Could you check a few things on this drawing? It's one solid part, dimensions in mm from its lowest x, y, z. Give positions to 0.01 mm unless a question says otherwise; leave off trailing zeros. Order: outer loops, then holes, each group sorted by start corner. A loop starts at its lowest first (then second) coordinate and runs counter-clockwise, first axis right, second up. Notation, with made-up numbers: (83.25, -6.75) - (100.25, -6.75) arc R30 ccw to (100.25, 28.25) - close; hole circle Ø9 at (60.5, 65). An arc over 180 degrees is marked (long way). Answer as CSV lines item,"result".
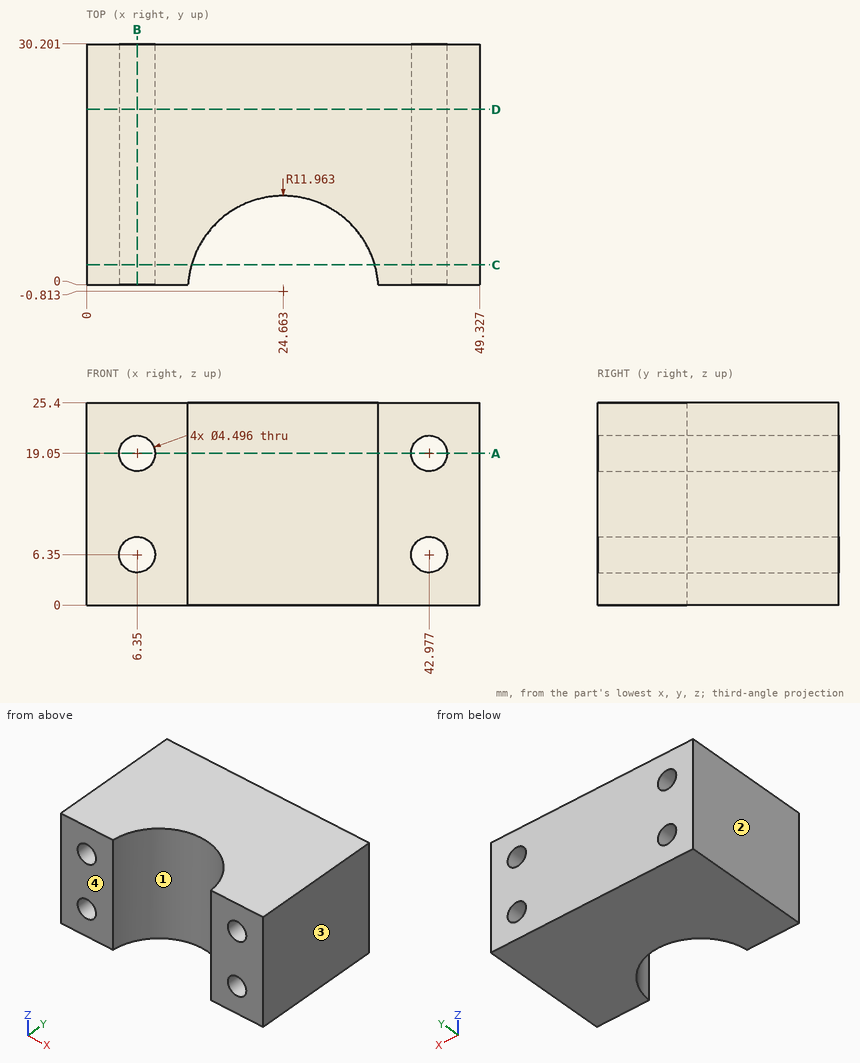
1) If we mould it in two halves opening along X, with no side actions, what happens to the marked faces 1, 2, 3 and 4? For each: +X half, -X half, draft (parallel to the pull), parting line (faces both ways), or undercut.
Answer block:
face 1,"undercut"
face 2,"-X half"
face 3,"+X half"
face 4,"draft"
2) I want a section at C-C on y = 2.5. Write out the boundary of the cut face in (x, z).
Answer block:
outline,"(0, 0) - (13.17, 0) - (13.17, 25.4) - (0, 25.4) - close; (36.16, 0) - (49.33, 0) - (49.33, 25.4) - (36.16, 25.4) - close; hole circle Ø4.5 at (6.35, 6.35); hole circle Ø4.5 at (6.35, 19.05); hole circle Ø4.5 at (42.98, 6.35); hole circle Ø4.5 at (42.98, 19.05)"
3) I'm going to push flat-ended pins straight in: P1, Ø1.5, axis at x = 22.5, z = 22.5, coming from the -Y side; P2, Ø3.5, axis at x = 42.98, z = 19.05, coming from the +Y side. Where does each tip first touch, or does it pass through?
Answer block:
P1,"y = 10.79"
P2,"through"
4) I need wall thicknesses on line 1 along Z through (x, y) = (6.35, 11); line 2 along Z through (x, y) = (45, 16.5); line 3 along X through (y, z) = (2.5, 10). Which ranges of each line are inside material? Lowest first, please. Write a range as [from, to].
Answer block:
line 1,"[0, 4.1], [8.6, 16.8], [21.3, 25.4]"
line 2,"[0, 5.37], [7.33, 18.07], [20.03, 25.4]"
line 3,"[0, 13.17], [36.16, 49.33]"
5) I want a section at B-B on x = 6.35. Write out the boundary of the cut face in (y, z).
Answer block:
outline,"(0, 0) - (30.2, 0) - (30.2, 4.1) - (0, 4.1) - close; (0, 8.6) - (30.2, 8.6) - (30.2, 16.8) - (0, 16.8) - close; (0, 21.3) - (30.2, 21.3) - (30.2, 25.4) - (0, 25.4) - close"
6) I want a section at D-D on y = 22. Write out the boundary of the cut face in (x, z), plus the area to 3 significant figures.
Answer block:
outline,"(0, 0) - (49.33, 0) - (49.33, 25.4) - (0, 25.4) - close; hole circle Ø4.5 at (6.35, 6.35); hole circle Ø4.5 at (6.35, 19.05); hole circle Ø4.5 at (42.98, 6.35); hole circle Ø4.5 at (42.98, 19.05)"
area,"1,190 mm2"
7) I want a section at A-A on z = 19.05. Write out the boundary of the cut face in (x, y) (1 decimal).
Answer block:
outline,"(0, 0) - (4.1, 0) - (4.1, 30.2) - (0, 30.2) - close; (8.6, 0) - (12.7, 0) arc R12 cw to (36.6, 0) - (40.7, 0) - (40.7, 30.2) - (8.6, 30.2) - close; (45.2, 0) - (49.3, 0) - (49.3, 30.2) - (45.2, 30.2) - close"
